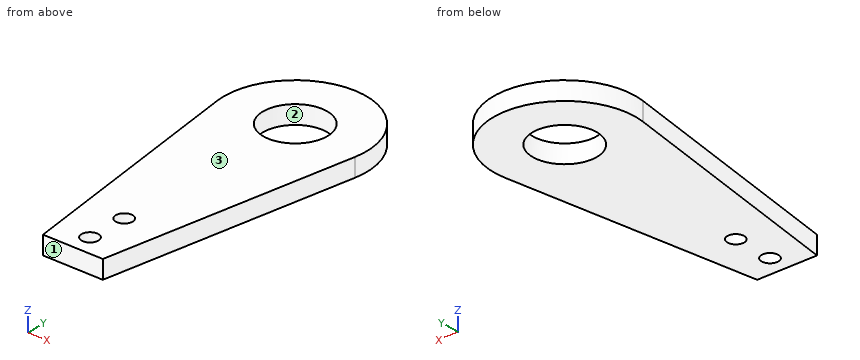
```python
from build123d import *

# Parameters (mm, degrees)
SKETCH1_R           = 2.075
SKETCH1_R_2         = 7.8875
BOSS_EXTRUDE2_DEPTH = 4.5


with BuildPart() as part:
    # Sketch1 → Boss-Extrude2 (new body)
    with BuildSketch(Plane.XY):
        with BuildLine():
            Line((-7.5, -5), (7.5, -5))
            Line((7.5, -5), (17.287829772, 57.283211128))
            ThreePointArc((17.287829772, 57.283211128), (0, 77.5), (-17.287829772, 57.283211128))
            Line((-17.287829772, 57.283211128), (-7.5, -5))
        make_face()
        Circle(SKETCH1_R, mode=Mode.SUBTRACT)
        with Locations((0, 60)):
            Circle(SKETCH1_R_2, mode=Mode.SUBTRACT)
        with Locations((0, 10)):
            Circle(SKETCH1_R, mode=Mode.SUBTRACT)
    extrude(amount=BOSS_EXTRUDE2_DEPTH)


solid = part.part
```
The listing builds one solid part. Answer for the finished solid, in the listing's coordinates (mm). Face numbers are marked on the shaded views. Coordinates: 2 decimals unless noted, no trailing zeros. Write each loop counter-clockwise with the first axis right and the second up, starting at its lowest first coordinate (ties: lowest second). Pieces come first, ordered by that corner, then holes.
Q1. Section A-A, the plane y = 60 is taken. Write down the section's boundary in (x, z).
Returned:
outline: (-17.5, 0) - (-7.89, 0) - (-7.89, 4.5) - (-17.5, 4.5) - close; (7.89, 0) - (17.5, 0) - (17.5, 4.5) - (7.89, 4.5) - close
Q2. Section C-C, the plane z = 2.35 is taken. Give the number of separate pieces and of enclosed holes in the cut face, then the cut area to 3 significant figures.
Returned:
separate pieces: 1
enclosed holes: 3
area: 1,900 mm2
Q3. The mould has two halves that part along Y. Classify the marked faces 1, 2 and 3: released by +Y, released by -Y, zero draft, split by the parting line, or undercut.
Returned:
face 1: released by -Y
face 2: undercut
face 3: zero draft
Q4. Section B-B, the plane x = 0 is taken. Write down the section's boundary in (y, z) (1 decimal), then the cut area to 3 significant figures.
Returned:
outline: (-5, 0) - (-2.1, 0) - (-2.1, 4.5) - (-5, 4.5) - close; (2.1, 0) - (7.9, 0) - (7.9, 4.5) - (2.1, 4.5) - close; (12.1, 0) - (52.1, 0) - (52.1, 4.5) - (12.1, 4.5) - close; (67.9, 0) - (77.5, 0) - (77.5, 4.5) - (67.9, 4.5) - close
area: 263 mm2
Q5. Find the intervals of material crossed by line 1 along Y through (x, z) = (0.5, 4.3); line 2 along X through (y, z) = (-1, 1.05); line 3 along X through (y, z) = (54.5, 2.7), in increasing order.
Returned:
line 1: y = -5 to -2.01, 2.01 to 7.99, 12.01 to 52.13, 67.87 to 77.49
line 2: x = -8.13 to -1.82, 1.82 to 8.13
line 3: x = -16.85 to -5.65, 5.65 to 16.85
Q6. Given P1, Ø2, axis at x = -6.5, z = 3.5, coming from the +Y side; P2, Ø1.5, axis at y = 25.5, z = 2.5, coming from the +X side; P3, Ø4, axis at x = -11.5, y = 17, coming from the -Z side, each flat-ended and moving along its own axis, determine where each tip first touches the part or whether it passes through.
Returned:
P1: stops at y = 76.61
P2: stops at x = 12.41
P3: stops at z = 0
Q7. Section D-D, the plane x = 4 is taken. Write down the section's boundary in (y, z).
Returned:
outline: (-5, 0) - (53.2, 0) - (53.2, 4.5) - (-5, 4.5) - close; (66.8, 0) - (77.04, 0) - (77.04, 4.5) - (66.8, 4.5) - close
